Geometry check sheet. Reference: the model listing, model coordinates, mm. A direction names the side the tool comes from. Coordinates: 2 decimals unless noted, no trailing zeros. Loops run counter-clockwise (first coordinate to the right, second up) from the corner with the lowest first, then second, coordinate; pieces in that order, holes last. Notation, with made-up numbers: M 72,87 L 93,87 A5 ccw 93,95 Z; hole C 38.5,43 d1. An arc over 180 degrees is marked long. Use CSV: the item, a comma, the result in double quotes.
```python
from build123d import *

# Parameters (mm, degrees)
SKETCH1_R           = 11.1125
BOSS_EXTRUDE1_DEPTH = 66.675
SKETCH2_W           = 15.875
SKETCH2_H           = 11.1125
BOSS_EXTRUDE2_DEPTH = 12.7
SKETCH3_R           = 4.7625
BOSS_EXTRUDE3_DEPTH = 12.7


with BuildPart() as part:
    # Sketch1 → Boss-Extrude1 (new body)
    with BuildSketch(Plane(origin=(0, 0, 0), x_dir=(1, 0, 0), z_dir=(0, 1, 0))):
        with Locations(Location((0, 0, 0), (0, 0, 270))):
            Circle(SKETCH1_R)
    extrude(amount=BOSS_EXTRUDE1_DEPTH)

    # Sketch2 → Boss-Extrude2 (add)
    with BuildSketch(Plane.XY):
        with Locations((0, 5.55625)):
            Rectangle(SKETCH2_W, SKETCH2_H)
    extrude(amount=BOSS_EXTRUDE2_DEPTH)

    # Sketch3 → Boss-Extrude3 (add)
    with BuildSketch(Plane(origin=(0, 66.675, 0), x_dir=(1, 0, 0), z_dir=(0, 1, 0))):
        with Locations(Location((0, 0, 0), (0, 0, 270))):
            Circle(SKETCH3_R)
    extrude(amount=BOSS_EXTRUDE3_DEPTH)


solid = part.part
```
1. Section check C-C, the plane y = 51. Record the cut outline in (x, z) (1 decimal).
The answers:
outline,"C 0,0 d22.2"
2. Gauge pin test, flat ends, axial feed: P1, Ø1.5, axis at x = 2.5, z = 7, coming from the -Y side; P2, Ø5.5, axis at x = 3, z = 9.5, coming from the +Y side (3 decimals); P3, Ø2, axis at x = -6, y = 25, coming from the +Z side; P4, Ø1.5, axis at y = 7, z = 10.5, coming from the -X side. Record the tip position at first contact, or that the pin passes through.
The answers:
P1,"y = 0"
P2,"y = 66.675"
P3,"z = 9.92"
P4,"x = -7.94"
3. Section check B-B, the plane z = 3.25. Record the cut outline in (x, y) (3 decimals).
The answers:
outline,"M -10.627,0 L 10.627,0 L 10.627,66.675 L 3.481,66.675 L 3.481,79.375 L -3.481,79.375 L -3.481,66.675 L -10.627,66.675 Z"
4. Thickness scan on line 1 (X direction, y = 9, z = 11); line 2 (Y direction, x = 6.5, z = 6.25) (3 decimals); line 3 (X direction, y = 66.5, z = -0.5). Record the ranges inside material, lowest first. Write a range as [from, to].
The answers:
line 1,"[-7.94, 7.94]"
line 2,"[0, 66.675]"
line 3,"[-11.1, 11.1]"
5. Set-up check for faces 1 (the flat face through (-0.1, 11.112, 11.3)), 2 (the flat face through (7.938, 5, 10)), 3 (the flat face through (-7.938, 5, 10)), 4 (the flat face through (0, 6, 12.7)), 5 (the flat face through (-5, 66.675, 0)): record each of +Z, -Z, +X, -X, +Y, -Y from which the full face is reachable in a straight line by a thin tool's end or side.
The answers:
face 1,"+Z, +Y"
face 2,"+Z, +X, +Y, -Y"
face 3,"+Z, -X, +Y, -Y"
face 4,"+Z, +X, -X, +Y, -Y"
face 5,"+Y"
6. Section check D-D, the plane z = 0. Record the cut outline in (x, y) (1 decimal).
The answers:
outline,"M -11.1,0 L 11.1,0 L 11.1,66.7 L 4.8,66.7 L 4.8,79.4 L -4.8,79.4 L -4.8,66.7 L -11.1,66.7 Z"
7. Section check A-A, the plane x = 0. Record the cut outline in (y, z) (1 decimal), plus the area to 3 significant figures.
The answers:
outline,"M 0,-11.1 L 66.7,-11.1 L 66.7,-4.8 L 79.4,-4.8 L 79.4,4.8 L 66.7,4.8 L 66.7,11.1 L 11.1,11.1 L 11.1,12.7 L 0,12.7 Z"
area,"1,620 mm^2"
